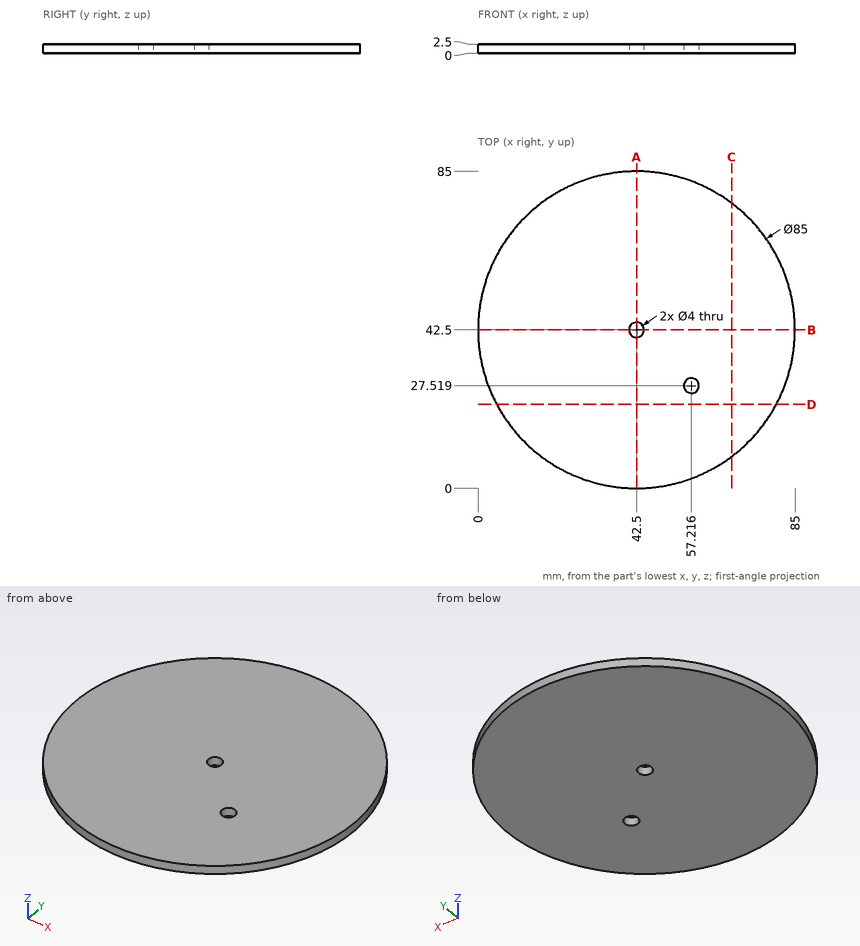
Design review of the part shown in the three views and the two pictorial views. Dimensions are in mm from the part's minimum x, y and z. Round coordinates to 2 decimals unless told otherwise and drop trailing zeros. Write each loop counter-clockwise with the first axis right and the second up, starting at its lowest first coordinate (ties: lowest second). Pieces come first, ordered by that corner, then holes. Notation, with made-up numbers: (-39, -21) -> (19, -21) arc R24 cw to (19, -11) -> close; hole circle Ø11 at (31, 64.5). An arc over 180 degrees is marked (long way). One line per question, with ' | ' between items. Start each with the question number.
1) Add section D-D (y = 22.5). Write out the cut boundary in (x, z).
2) Add section C-C (x = 68). Write out the cut boundary in (y, z), and give its area (3 significant figures).
3) For pin 1 Ø2.5 at (x, y) = (57.22, 27.52) entering from -Z; pin 2 Ø1.5 at (y, z) = (12, 2) entering from +X; pin 3 Ø1 at (y, z) = (64.5, 2) entering from +X, all flat-tipped, find the tip position at first contact; note any pin that passes through.
4) Add section A-A (x = 42.5). Write out the cut boundary in (y, z).
5) Wall thickness on line 1 along Y through (x, z) = (42.5, 1.35); line 2 along X through (y, z) = (43, 0.65); line 3 along Y through (x, z) = (57.5, 1) (1 decimal): over which ranges is each line inside the solid? List them lowest first.
Reported:
1) outline: (5, 0) -> (80, 0) -> (80, 2.5) -> (5, 2.5) -> close
2) outline: (8.5, 0) -> (76.5, 0) -> (76.5, 2.5) -> (8.5, 2.5) -> close | area: 170 mm²
3) pin 1: passes through | pin 2: stops at x = 72.85 | pin 3: stops at x = 79.16
4) outline: (0, 0) -> (40.5, 0) -> (40.5, 2.5) -> (0, 2.5) -> close; (44.5, 0) -> (85, 0) -> (85, 2.5) -> (44.5, 2.5) -> close
5) line 1: y = 0 to 40.5, 44.5 to 85 | line 2: x = 0 to 40.56, 44.44 to 85 | line 3: y = 2.7 to 25.5, 29.5 to 82.3
